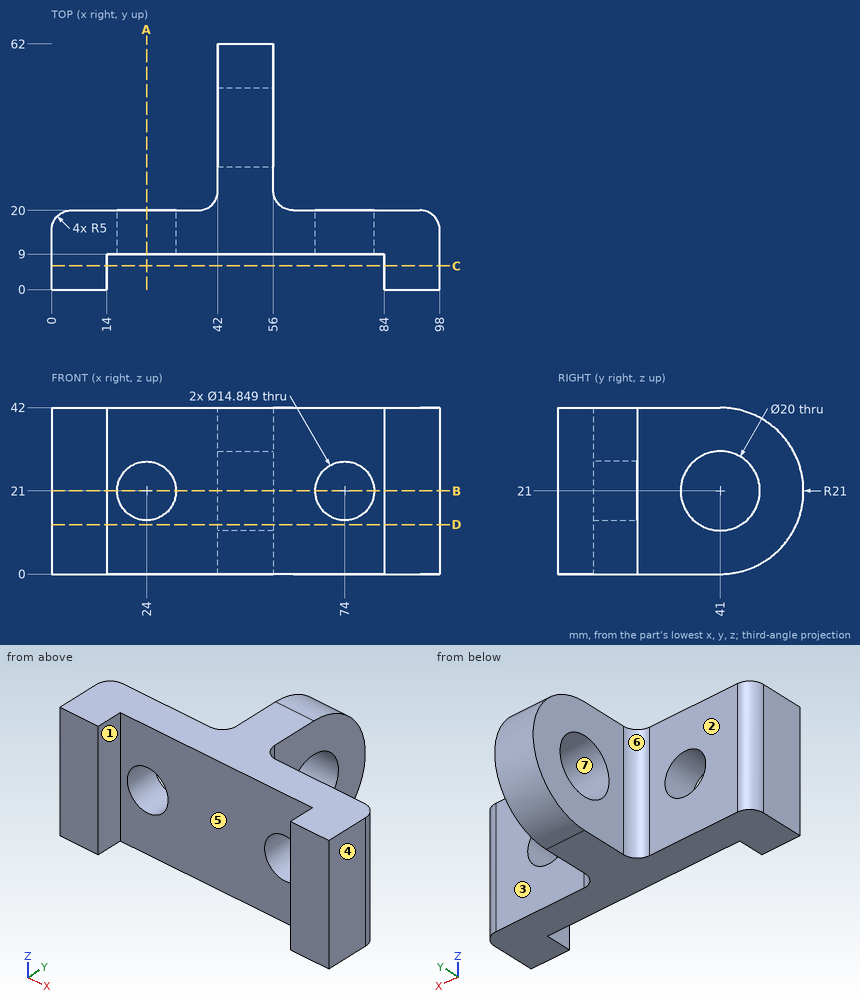
Job drawing, mm, ordinate dimensions from the low corner. One solid piece. A direction names the side the tool comes from. Give positions to 0.01 mm unless a question says otherwise; leave off trailing zeros. Order: outer loops, then holes, each group sorted by start corner. A loop starts at its lowest first (then second) coordinate and runs counter-clockwise, first axis right, second up. Notation, with made-up numbers: (87, 27.5) - (115, 27.5) arc R30 cw to (115, 62.5) - close; hole circle Ø5 at (0, 87.25). An arc over 180 degrees is marked (long way). Answer in a Markdown table with one row per item.
1. Saw through at B-B, the plane z = 21. Give the cut face in (x, y) (1 decimal), plus the area to 3 significant figures.
Data:
| item | result |
|---|---|
| outline | (0, 0) - (14, 0) - (14, 9) - (16.6, 9) - (16.6, 20) - (5, 20) arc R5 ccw to (0, 15) - close; (31.4, 9) - (66.6, 9) - (66.6, 20) - (61, 20) arc R5 cw to (56, 25) - (56, 31) - (42, 31) - (42, 25) arc R5 cw to (37, 20) - (31.4, 20) - close; (42, 51) - (56, 51) - (56, 62) - (42, 62) - close; (81.4, 9) - (84, 9) - (84, 0) - (98, 0) - (98, 15) arc R5 ccw to (93, 20) - (81.4, 20) - close |
| area | 1,310 mm² |
2. Probe probe 1 along X at (y, z) = (14, 21) (1 decimal); probe 2 along Y at (x, z) = (52, 21); probe 3 along X at (y, z) = (8, 20). List the from-to ranges inside material, lowest first. Write a range as [from, to].
Data:
| item | result |
|---|---|
| probe 1 | x = [0, 16.6], [31.4, 66.6], [81.4, 98] |
| probe 2 | y = [9, 31], [51, 62] |
| probe 3 | x = [0, 14], [84, 98] |
3. Flat gauge pins, fed straight in: pin 1 (18.5 mm diameter, centred on y = 34.5, z = 20, fed in from -X); pin 2 (5 mm diameter, centred on x = 41, z = 17.5, fed in from +Y) (1 decimal); pin 3 (4 mm diameter, centred on x = 35, z = 22, fed in from -Y). Where does each tip first touch, or does it go through?
Data:
| item | result |
|---|---|
| pin 1 | stops at x = 42 |
| pin 2 | stops at y = 62 |
| pin 3 | stops at y = 9 |
4. Saw through at A-A, the plane x = 24. Give the cut face in (y, z) (1 decimal), plus the area to 3 significant figures.
Data:
| item | result |
|---|---|
| outline | (9, 0) - (20, 0) - (20, 13.6) - (9, 13.6) - close; (9, 28.4) - (20, 28.4) - (20, 42) - (9, 42) - close |
| area | 299 mm² |
5. Pull direction Y, two halves, no side cores. Call the marked faces 5, 6 and 7: pulls with the +Y half, pulls with the -Y half, needs draft (parallel to the pull), parting line crosses it, or undercut.
Data:
| item | result |
|---|---|
| face 5 | pulls with the -Y half |
| face 6 | pulls with the +Y half |
| face 7 | undercut |
6. Saw through at C-C, the plane y = 6. Give the cut face in (x, z), plus the area to 3 significant figures.
Data:
| item | result |
|---|---|
| outline | (0, 0) - (14, 0) - (14, 42) - (0, 42) - close; (84, 0) - (98, 0) - (98, 42) - (84, 42) - close |
| area | 1,180 mm² |
7. Tool access for the marked faces 1, 2, 3 and 4: list every direction of +Z, -Z, +X, -X, +Y, -Y with a clear straight run to the whole face (end or side of a thin tool).
Data:
| item | result |
|---|---|
| face 1 | +Z, -Z, -Y |
| face 2 | +Z, -Z, -X, +Y |
| face 3 | +Z, -Z, +X, +Y |
| face 4 | +Z, -Z, +X, +Y, -Y |
8. Saw through at D-D, the plane z = 12.5. Give the cut face in (x, y), plus the area to 3 significant figures.
Data:
| item | result |
|---|---|
| outline | (0, 0) - (14, 0) - (14, 9) - (84, 9) - (84, 0) - (98, 0) - (98, 15) arc R5 ccw to (93, 20) - (61, 20) arc R5 cw to (56, 25) - (56, 35.73) - (42, 35.73) - (42, 25) arc R5 cw to (37, 20) - (5, 20) arc R5 ccw to (0, 15) - close; (42, 46.27) - (56, 46.27) - (56, 60.2) - (42, 60.2) - close |
| area | 1,750 mm² |
